```python
from build123d import *

# Parameters (mm, degrees)
SKETCH1_W               = 25
SKETCH1_H               = 39
SKETCH1_W_2             = 21
SKETCH1_H_2             = 35
BOSS_EXTRUDE1_DEPTH     = 30
SKETCH1_2_W             = 25
SKETCH1_2_H             = 39
SKETCH1_2_W_2           = 21
SKETCH1_2_H_2           = 35
BOSS_EXTRUDE2_DEPTH     = 5
CUT_EXTRUDE1_DEPTH      = 38.901187316
CUT_EXTRUDE1_DEPTH_BACK = 38.901187316
SKETCH4_R               = 2.75


with BuildPart() as part:
    # Sketch1 → Boss-Extrude1 (new body)
    with BuildSketch(Plane(origin=(0, 0, 0), x_dir=(1, 0, 0), z_dir=(0, 1, 0))):
        Rectangle(SKETCH1_W, SKETCH1_H)
        Rectangle(SKETCH1_W_2, SKETCH1_H_2, mode=Mode.SUBTRACT)
    extrude(amount=BOSS_EXTRUDE1_DEPTH)

    # Sketch1_2 → Boss-Extrude2 (add)
    # profile 1 of 2: a face of its own
    with BuildSketch(Plane(origin=(0, 0, 0), x_dir=(1, 0, 0), z_dir=(0, 1, 0))):
        Rectangle(SKETCH1_2_W, SKETCH1_2_H)
        Rectangle(SKETCH1_2_W_2, SKETCH1_2_H_2, mode=Mode.SUBTRACT)
    # profile 2 of 2: a face of its own
    with BuildSketch(Plane(origin=(0, 0, 0), x_dir=(1, 0, 0), z_dir=(0, 1, 0))):
        Rectangle(SKETCH1_2_W_2, SKETCH1_2_H_2)
    extrude(amount=-BOSS_EXTRUDE2_DEPTH)

    # Sketch4 → Cut-Extrude1 (cut, two sides: drawn at the far end of the back side and taken through both)
    with BuildSketch(Plane(origin=(0, 0, 0), x_dir=(1, 0, 0), z_dir=(0, 1, 0)).offset(-CUT_EXTRUDE1_DEPTH_BACK)):
        with Locations(Location((0, 0, 0), (0, 0, 270))):
            Circle(SKETCH4_R)
    extrude(amount=CUT_EXTRUDE1_DEPTH + CUT_EXTRUDE1_DEPTH_BACK, mode=Mode.SUBTRACT)


solid = part.part
```
Geometry check sheet. Reference: the model listing, model coordinates, mm. A direction names the side the tool comes from. Coordinates: 2 decimals unless noted, no trailing zeros. Order: outer loops, then holes, each group sorted by start corner. A loop starts at its lowest first (then second) coordinate and runs counter-clockwise, first axis right, second up. Notation, with made-up numbers: (-27.5, 50) - (26.5, 50) arc R31 ccw to (26.5, 74) - close; hole circle Ø2 at (-27, 83). An arc over 180 degrees is marked (long way). Answer as a JSON object with one key per item and string values. Group by question number.
Item 1: Tool access check on faces 4 (the face through (0, 0, -4)), 5 (the face through (-2.685, -2.535, -0.596)). Record the directions out of +Z, -Z, +X, -X, +Y, -Y that give a thin tool (end or side, any length) a straight path to the whole face; none if there is none.
Item 2: Depth check by flat-ended pin: pin 1 Ø3.5 at (x, z) = (0, 0) entering from -Y. Enter the tip coordinate at first touch or a pass-through.
Item 3: Sectioned sample at B-B, the plane x = 0. Record the cut outline in (y, z), and give its area (4 significant figures).
Item 4: Scan lines: probe 1 along Z at (x, y) = (-6, 15); probe 2 along Z at (x, y) = (0, -1.55); probe 3 along X at (y, z) = (3, -5.5). Record each from-to range of solid material in increasing order.
Item 5: Sectioned sample at D-D, the plane x = -3.75. Record the cut outline in (y, z), and give its area (3 significant figures).
Item 6: Sectioned sample at C-C, the plane y = 21.5. Record the cut outline in (x, z), and give its area (3 significant figures).
Item 7: Sectioned sample at A-A, the plane z = 0. Record the cut outline in (x, y), and give its area (4 significant figures).
Item 8: Draft check along X on faces 1 (the face through (12.5, 13, 0)), 2 (the face through (-10.5, 15, 0)), 3 (the face through (0, 13, -19.5)). Enter one of: +X half, -X half, draft (parallel to the pull), parting line (faces both ways), or undercut.
Resolved:
{
 "1": {"face 4": "+Y", "face 5": "+Y, -Y"},
 "2": {"pin 1": "through"},
 "3": {"outline": "(-5, -19.5) - (30, -19.5) - (30, -17.5) - (0, -17.5) - (0, -2.75) - (-5, -2.75) - close; (-5, 2.75) - (0, 2.75) - (0, 17.5) - (30, 17.5) - (30, 19.5) - (-5, 19.5) - close", "area": "287.5 mm^2"},
 "4": {"probe 1": "-19.5 to -17.5, 17.5 to 19.5", "probe 2": "-19.5 to -2.75, 2.75 to 19.5", "probe 3": "-12.5 to -10.5, 10.5 to 12.5"},
 "5": {"outline": "(-5, -19.5) - (30, -19.5) - (30, -17.5) - (0, -17.5) - (0, 17.5) - (30, 17.5) - (30, 19.5) - (-5, 19.5) - close", "area": "315 mm^2"},
 "6": {"outline": "(-12.5, -19.5) - (12.5, -19.5) - (12.5, 19.5) - (-12.5, 19.5) - close; hole (-10.5, -17.5) - (10.5, -17.5) - (10.5, 17.5) - (-10.5, 17.5) - close", "area": "240 mm^2"},
 "7": {"outline": "(-12.5, -5) - (-2.75, -5) - (-2.75, 0) - (-10.5, 0) - (-10.5, 30) - (-12.5, 30) - close; (2.75, -5) - (12.5, -5) - (12.5, 30) - (10.5, 30) - (10.5, 0) - (2.75, 0) - close", "area": "217.5 mm^2"},
 "8": {"face 1": "+X half", "face 2": "undercut", "face 3": "draft"}
}
